Source: CAD feature listing. Evaluate the final solid. Frame: model axes, mm. Coordinates: 2 decimals unless noted, no trailing zeros. Order: outer loops, then holes, each group sorted by start corner. A loop starts at its lowest first (then second) coordinate and runs counter-clockwise, first axis right, second up. Notation, with made-up numbers: (31, -1.75) -> (65, -1.75) arc R27 cw to (65, 35.25) -> close; hole circle Ø1 at (-22, 74). An arc over 180 degrees is marked (long way). Write each question's results on one line, items separated by ' | '. Start each with the question number.
from build123d import *

# Parameters (mm, degrees)
SKETCH_1_R          = 2.2
EXTRUDE_1_DEPTH     = 5
FILLET_1_R          = 10
CUT_EXTRUDE_1_REACH = 317.85
SKETCH_2_R          = 2.2


with BuildPart() as part:
    # 草图1 → 凸台-拉伸1 (new body)
    with BuildSketch(Plane.XY):
        Polygon((-51.5, 7), (-51.5, -163), (46.5, -163), (46.5, -218), (130.5, -218), (130.5, -163), (228.5, -163), (228.5, 7), (130.5, 7), (130.5, 62), (46.5, 62), (46.5, 7), align=None)
        with Locations((-15, -143.9)):
            Circle(SKETCH_1_R, mode=Mode.SUBTRACT)
        with Locations((15, -143.9)):
            Circle(SKETCH_1_R, mode=Mode.SUBTRACT)
        with Locations((-15, -114.1)):
            Circle(SKETCH_1_R, mode=Mode.SUBTRACT)
        with Locations((15, -114.1)):
            Circle(SKETCH_1_R, mode=Mode.SUBTRACT)
        with Locations((162, -143.9)):
            Circle(SKETCH_1_R, mode=Mode.SUBTRACT)
        with Locations((192, -143.9)):
            Circle(SKETCH_1_R, mode=Mode.SUBTRACT)
        with Locations((162, -114.1)):
            Circle(SKETCH_1_R, mode=Mode.SUBTRACT)
        with Locations((192, -114.1)):
            Circle(SKETCH_1_R, mode=Mode.SUBTRACT)
        with Locations((-15, -41.9)):
            Circle(SKETCH_1_R, mode=Mode.SUBTRACT)
        with Locations((15, -41.9)):
            Circle(SKETCH_1_R, mode=Mode.SUBTRACT)
        with Locations((-15, -12.1)):
            Circle(SKETCH_1_R, mode=Mode.SUBTRACT)
        with Locations((15, -12.1)):
            Circle(SKETCH_1_R, mode=Mode.SUBTRACT)
        with Locations((162, -41.9)):
            Circle(SKETCH_1_R, mode=Mode.SUBTRACT)
        with Locations((192, -41.9)):
            Circle(SKETCH_1_R, mode=Mode.SUBTRACT)
        with Locations((162, -12.1)):
            Circle(SKETCH_1_R, mode=Mode.SUBTRACT)
        with Locations((192, -12.1)):
            Circle(SKETCH_1_R, mode=Mode.SUBTRACT)
    extrude(amount=EXTRUDE_1_DEPTH)

    # 圆角1
    fillet_1_edges = [part.edges().sort_by_distance(p)[0] for p in [
        (130.5, 7, 2.5),
        (228.5, 7, 2.5),
        (228.5, -163, 2.5),
        (130.5, -163, 2.5),
        (130.5, -218, 2.5),
        (46.5, -218, 2.5),
        (46.5, -163, 2.5),
        (-51.5, -163, 2.5),
        (-51.5, 7, 2.5),
        (46.5, 7, 2.5),
        (46.5, 62, 2.5),
        (130.5, 62, 2.5),
    ]]
    fillet(fillet_1_edges, radius=FILLET_1_R)

    # 草图2 → 切除-拉伸1 (cut, up to next)
    with BuildSketch(Plane(origin=(0, 0, 0), x_dir=(-1, 0, 0), z_dir=(0, 0, -1)), mode=Mode.PRIVATE) as cut_extrude_1_sk1:
        with Locations(Location((-64.458980338, -103.063390978, 0), (0, 0, 90))):
            Circle(SKETCH_2_R)
    cut_extrude_1_tool1 = extrude(cut_extrude_1_sk1.sketch, amount=-CUT_EXTRUDE_1_REACH, mode=Mode.PRIVATE) & part.part
    # 草图2 → 切除-拉伸1 (cut, up to next)
    with BuildSketch(Plane(origin=(0, 0, 0), x_dir=(-1, 0, 0), z_dir=(0, 0, -1)), mode=Mode.PRIVATE) as cut_extrude_1_sk2:
        with Locations(Location((-34.458980337, -135.063390978, 0), (0, 0, 90))):
            Circle(SKETCH_2_R)
    cut_extrude_1_tool2 = extrude(cut_extrude_1_sk2.sketch, amount=-CUT_EXTRUDE_1_REACH, mode=Mode.PRIVATE) & part.part
    # 草图2 → 切除-拉伸1 (cut, up to next)
    with BuildSketch(Plane(origin=(0, 0, 0), x_dir=(-1, 0, 0), z_dir=(0, 0, -1)), mode=Mode.PRIVATE) as cut_extrude_1_sk3:
        with Locations(Location((-64.458980338, -167.063390978, 0), (0, 0, 90))):
            Circle(SKETCH_2_R)
    cut_extrude_1_tool3 = extrude(cut_extrude_1_sk3.sketch, amount=-CUT_EXTRUDE_1_REACH, mode=Mode.PRIVATE) & part.part
    add(cut_extrude_1_tool1.solids().sort_by_distance((64.45898, -103.063391, 0))[0], mode=Mode.SUBTRACT)
    add(cut_extrude_1_tool2.solids().sort_by_distance((34.45898, -135.063391, 0))[0], mode=Mode.SUBTRACT)
    add(cut_extrude_1_tool3.solids().sort_by_distance((64.45898, -167.063391, 0))[0], mode=Mode.SUBTRACT)


solid = part.part
(1) Line query: L1, parallel to Y at x = 15, z = 1.15; L2, parallel to X at y = -42, z = 2.6; L3, parallel to Y at x = 193.5, z = 0.9. Output: solid intervals per line, ascending.
(2) Section B-B on x = 22.5. Return the cut outline in (y, z).
(3) Section C-C on z = 2.75. Count the separate pieces of the cut face and the enclosed holes in it, then the cut area to 3 significant figures.
(4) Section A-A on y = 45.5. Return the cut outline in (x, z), then the cut area to 3 significant figures.
Results list:
1) L1: y = -163 to -146.1, -141.7 to -116.3, -111.9 to -44.1, -39.7 to -14.3, -9.9 to 7 | L2: x = -51.5 to -17.2, -12.8 to 12.8, 17.2 to 159.8, 164.2 to 189.8, 194.2 to 228.5 | L3: y = -163 to -145.51, -142.29 to -115.71, -112.49 to -43.51, -40.29 to -13.71, -10.49 to 7
2) outline: (-163, 0) -> (7, 0) -> (7, 5) -> (-163, 5) -> close
3) separate pieces: 1 | enclosed holes: 19 | area: 56,500 mm²
4) outline: (46.5, 0) -> (130.5, 0) -> (130.5, 5) -> (46.5, 5) -> close | area: 420 mm²
